The listing builds one solid part. Answer for the finished solid, in the listing's coordinates (mm). A direction names the side the tool comes from. Coordinates: 2 decimals unless noted, no trailing zeros. Write each loop counter-clockwise with the first axis right and the second up, starting at its lowest first coordinate (ties: lowest second). Pieces come first, ordered by that corner, then holes.
(1) For a pull along X with two mould halves and no side action, classify faces 1 (the cylindrical face through (-48.857, 32.29, 11.339)), 2 (the flat face through (-71, 27.036, -2)), 3 (the flat face through (-51.53, 29, -2)) as +X half, -X half, draft (parallel to the pull), parting line (faces both ways), or undercut.
(2) The part is cut by section B-B on y = 20.25. Determine the outline of the cut face in (x, z), plus the area to 3 significant figures.
(3) Which of the six approach directions +Z, -Z, +X, -X, +Y, -Y give full straight-line access (tool end or side, diameter ignored) to faces 4 (the flat face through (-57, 38, 23)), 5 (the flat face through (-71.53, 29, -2)), 6 (the flat face through (-51, 27.036, -2)), 7 (the flat face through (-70.03, 29, -2)), 8 (the flat face through (-71, 30.036, -2))?
(4) The part is cut by section C-C on z = 22. Determine the outline of the cut face in (x, y), plus the area to 3 significant figures.
(5) Straight lines are drawn through the part: line 1 (Z direction, x = -61.5, y = 30); line 2 (Z direction, x = -56.5, y = 18.25); line 3 (Y direction, x = -55.75, z = 5). For each, find the intervals that lie inside material, in ascending order.
(6) The part is cut by section D-D on z = 25.5. Determine the outline of the cut face in (x, y), plus the area to 3 significant figures.
(7) Given P1, Ø1.5, axis at y = 28.5, z = -2.5, coming from the +X side; P2, Ø1, axis at x = -51.5, z = 15.5, coming from the +Y side; P3, Ø1, axis at x = -69.5, z = 5.5, coming from the -Y side, each flat-ended and moving along its own axis, determine where each tip first touches the part or whether it passes through.
(8) The part is cut by section A-A on x = -52.75. Determine the outline of the cut face in (y, z).
from build123d import *

# Parameters (mm, degrees)
ESQUISSE1_R        = 12.5
BOSS_EXTRU_1_DEPTH = 23
ESQUISSE2_R        = 10
BOSS_EXTRU_2_DEPTH = 3
ESQUISSE3_R        = 1
BOSS_EXTRU_3_DEPTH = 5
ESQUISSE4_W        = 1.5
ESQUISSE4_H        = 3
BOSS_EXTRU_4_DEPTH = 4


with BuildPart() as part:
    # Esquisse1 → Boss.-Extru.1 (new body)
    with BuildSketch(Plane.XY):
        with Locations((-60.780131723, 28.535714286)):
            Circle(ESQUISSE1_R)
    extrude(amount=BOSS_EXTRU_1_DEPTH)

    # Esquisse2 → Boss.-Extru.2 (add)
    with BuildSketch(Plane.XY.offset(23)):
        with Locations((-60.780131723, 28.535714286)):
            Circle(ESQUISSE2_R)
    extrude(amount=BOSS_EXTRU_2_DEPTH)

    # Esquisse3 → Boss.-Extru.3 (add)
    with BuildSketch(Plane.XY.offset(26)):
        with Locations((-60.780131723, 28.535714286)):
            Circle(ESQUISSE3_R)
    extrude(amount=BOSS_EXTRU_3_DEPTH)

    # Esquisse4 → Boss.-Extru.4 (add)
    with BuildSketch(Plane(origin=(0, 0, 0), x_dir=(-1, 0, 0), z_dir=(0, 0, -1))):
        with Locations((70.780131723, 28.535714286)):
            Rectangle(ESQUISSE4_W, ESQUISSE4_H)
        with Locations((50.780131723, 28.535714286)):
            Rectangle(ESQUISSE4_W, ESQUISSE4_H)
    extrude(amount=BOSS_EXTRU_4_DEPTH)


solid = part.part
Model answer:
1. face 1: parting line
1. face 2: draft
1. face 3: undercut
2. outline: (-70.14, 0) - (-51.42, 0) - (-51.42, 23) - (-55.18, 23) - (-55.18, 26) - (-66.38, 26) - (-66.38, 23) - (-70.14, 23) - close
2. area: 464 mm2
3. face 4: +Z
3. face 5: -Z, -X, +Y, -Y
3. face 6: -Z, +X, -X, -Y
3. face 7: -Z, +Y, -Y
3. face 8: -Z, +X, -X, +Y
4. outline: circle Ø25 at (-60.78, 28.54)
4. area: 491 mm2
5. line 1: z = 0 to 26
5. line 2: z = 0 to 23
5. line 3: y = 17.09 to 39.98
6. outline: circle Ø20 at (-60.78, 28.54)
6. area: 314 mm2
7. P1: stops at x = -50.03
7. P2: stops at y = 37.43
7. P3: stops at y = 19.12
8. outline: (18.96, 0) - (38.12, 0) - (38.12, 23) - (34.5, 23) - (34.5, 26) - (22.58, 26) - (22.58, 23) - (18.96, 23) - close
